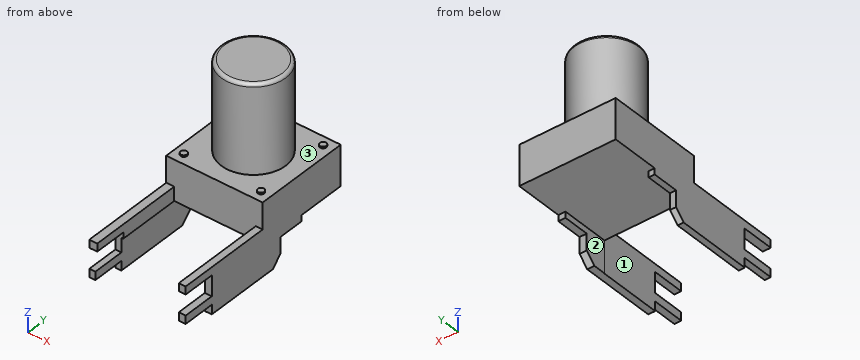
from build123d import *

# Parameters (mm, degrees)
SKETCH1_W               = 6
SKETCH1_H               = 6
BOSS_EXTRUDE1_DEPTH     = 2.5
SKETCH2_R               = 2
BOSS_EXTRUDE2_DEPTH     = 5.5
SKETCH3_R               = 0.2
BOSS_EXTRUDE3_DEPTH     = 0.1
BOSS_EXTRUDE4_DEPTH     = 6
SKETCH5_W               = 5.177961038
SKETCH5_H               = 4.130239003
CUT_EXTRUDE1_DEPTH      = 1
CUT_EXTRUDE1_DEPTH_BACK = 12.914158668
SKETCH6_W               = 5.072029737
SKETCH6_H               = 6.679255732
CUT_EXTRUDE2_DEPTH      = 8.131207494
CUT_EXTRUDE2_DEPTH_BACK = 3.853830155
FILLET1_R               = 0.2


with BuildPart() as part:
    # Sketch1 → Boss-Extrude1 (new body)
    with BuildSketch(Plane.XY):
        with Locations((3, 3)):
            Rectangle(SKETCH1_W, SKETCH1_H)
    extrude(amount=BOSS_EXTRUDE1_DEPTH)

    # Sketch3 → Boss-Extrude3 (add)
    with BuildSketch(Plane.XY.offset(2.5)):
        with Locations((0.598613773, 0.612952074)):
            Circle(SKETCH3_R)
        with Locations((5.401386227, 0.612952074)):
            Circle(SKETCH3_R)
        with Locations((5.401386227, 5.387047926)):
            Circle(SKETCH3_R)
        with Locations((0.598613773, 5.387047926)):
            Circle(SKETCH3_R)
    extrude(amount=BOSS_EXTRUDE3_DEPTH)



with BuildPart() as body_2:
    # Sketch2 → Boss-Extrude2 (new body)
    with BuildSketch(Plane.XY.offset(2.5)):
        with Locations((3, 3)):
            Circle(SKETCH2_R)
    extrude(amount=BOSS_EXTRUDE2_DEPTH)


with BuildPart() as part_1:
    add(part.part)

    add(body_2.part)  # Boss-Extrude4 merges body 2
    # Sketch4 → Boss-Extrude4 (add)
    with BuildSketch(Plane(origin=(6, 0, 0), x_dir=(0, 0, -1), z_dir=(1, 0, 0))):
        Polygon((-2.5, 3), (0.378290485, 3), (0.378290485, 1.362552045), (1.397956954, 1.362552045), (1.985037649, 0.77547135), (1.985037649, -3.91190451), (1.397956954, -3.91190451), (1.397956954, -5.914158668), (0.88812372, -5.914158668), (0.88812372, -3.91190451), (-0.379352601, -3.91190451), (-0.379352601, -5.914158668), (-0.868792506, -5.914158668), (-0.868792506, 0), (-2.5, 0), align=None)
    extrude(amount=-BOSS_EXTRUDE4_DEPTH)

    # Sketch5 → Cut-Extrude1 (cut, two sides)
    with BuildSketch(Plane(origin=(0, 6, 0), x_dir=(1, 0, 0), z_dir=(0, 1, 0))) as cut_extrude1_sk:
        with Locations((2.966920818, 2.065119502)):
            Rectangle(SKETCH5_W, SKETCH5_H)
    extrude(amount=CUT_EXTRUDE1_DEPTH, mode=Mode.SUBTRACT)
    extrude(cut_extrude1_sk.sketch, amount=-CUT_EXTRUDE1_DEPTH_BACK, mode=Mode.SUBTRACT)

    # Sketch6 → Cut-Extrude2 (cut, two sides)
    with BuildSketch(Plane.XY.offset(0.868792506)) as cut_extrude2_sk:
        with Locations((3.03473993, -3.339627866)):
            Rectangle(SKETCH6_W, SKETCH6_H)
    extrude(amount=CUT_EXTRUDE2_DEPTH, mode=Mode.SUBTRACT)
    extrude(cut_extrude2_sk.sketch, amount=-CUT_EXTRUDE2_DEPTH_BACK, mode=Mode.SUBTRACT)

    # Fillet1
    fillet1_edges = [part_1.edges().sort_by_distance(p)[0] for p in [
        (1, 3, 8),
    ]]
    fillet(fillet1_edges, radius=FILLET1_R)


solid = part_1.part
Build history of the part. All positions in model axes, mm. Face numbers are marked on the shaded views. A direction names the side the tool comes from. Round coordinates to 2 decimals unless told otherwise and drop trailing zeros. Write each loop counter-clockwise with the first axis right and the second up, starting at its lowest first coordinate (ties: lowest second). Pieces come first, ordered by that corner, then holes. Notation, with made-up numbers: (9, -1.75) -> (14, -1.75) arc R8 cw to (14, 8.25) -> close; hole circle Ø7 at (-21, 2). An arc over 180 degrees is marked (long way). Write item = value, one per line.
(1) Tool access for the marked faces 1, 2 and 3: list every direction of +Z, -Z, +X, -X, +Y, -Y with a clear straight run to the whole face (end or side of a thin tool).
Answer:
face_1 = +Z, -Z, -Y
face_2 = -Z, +Y, -Y
face_3 = +Z
(2) Band-saw the part on C-C (z = 4.5). Give the cut face in (x, y), then the cut area to 3 significant figures.
Answer:
outline = circle Ø4 at (3, 3)
area = 12.6 mm2
(3) Band-saw the part on B-B (x = 3). Give the cut face in (y, z), then the cut area to 3 significant figures.
Answer:
outline = (0, 0) -> (6, 0) -> (6, 2.5) -> (5, 2.5) -> (5, 7.8) arc R0.2 ccw to (4.8, 8) -> (1.2, 8) arc R0.2 ccw to (1, 7.8) -> (1, 2.5) -> (0, 2.5) -> close
area = 37.0 mm2
(4) Band-saw the part on A-A (y = -3.75). Give the cut face in (x, z), then the cut area to 3 significant figures.
Answer:
outline = (0, -1.99) -> (0.38, -1.99) -> (0.38, 0) -> (0.5, 0) -> (0.5, 0.87) -> (0, 0.87) -> close; (5.57, -1.99) -> (6, -1.99) -> (6, 0.87) -> (5.57, 0.87) -> close
area = 2.41 mm2
(5) Probe L1, parallel to X at y = -3, z = -0.75; L2, parallel to Z at x = 2.7, y = 5.5; L3, parallel to Z at x = 5.4, y = 0.5. List the from-to ranges inside material, lowest first.
Answer:
L1 = 0 to 0.38, 5.57 to 6
L2 = 0 to 2.5
L3 = 0 to 2.6
(6) Flat gauge pins, fed straight in: pin 1 (1.5 mm diameter, centred on x = 2, y = -0.5, fed in from -Z); pin 2 (2 mm diameter, centred on x = 4.5, y = -0.5, fed in from +Z); pin 3 (0.5 mm diameter, centred on x = 6, z = -1, fed in from +Y). Where does each tip first touch, or does it go through?
Answer:
pin_1 = 0
pin_2 = 2.5
pin_3 = 1.36
